Input: dimensioned drawing with shaded views. Units: mm. Origin: part minimum x, y, z. A direction names the side the tool comes from. Give positions to 0.01 mm unless a question says otherwise; leave off trailing zeros. Write each loop counter-clockwise with the first axis right and the second up, starting at its lowest first coordinate (ties: lowest second). Pieces come first, ordered by that corner, then holes.
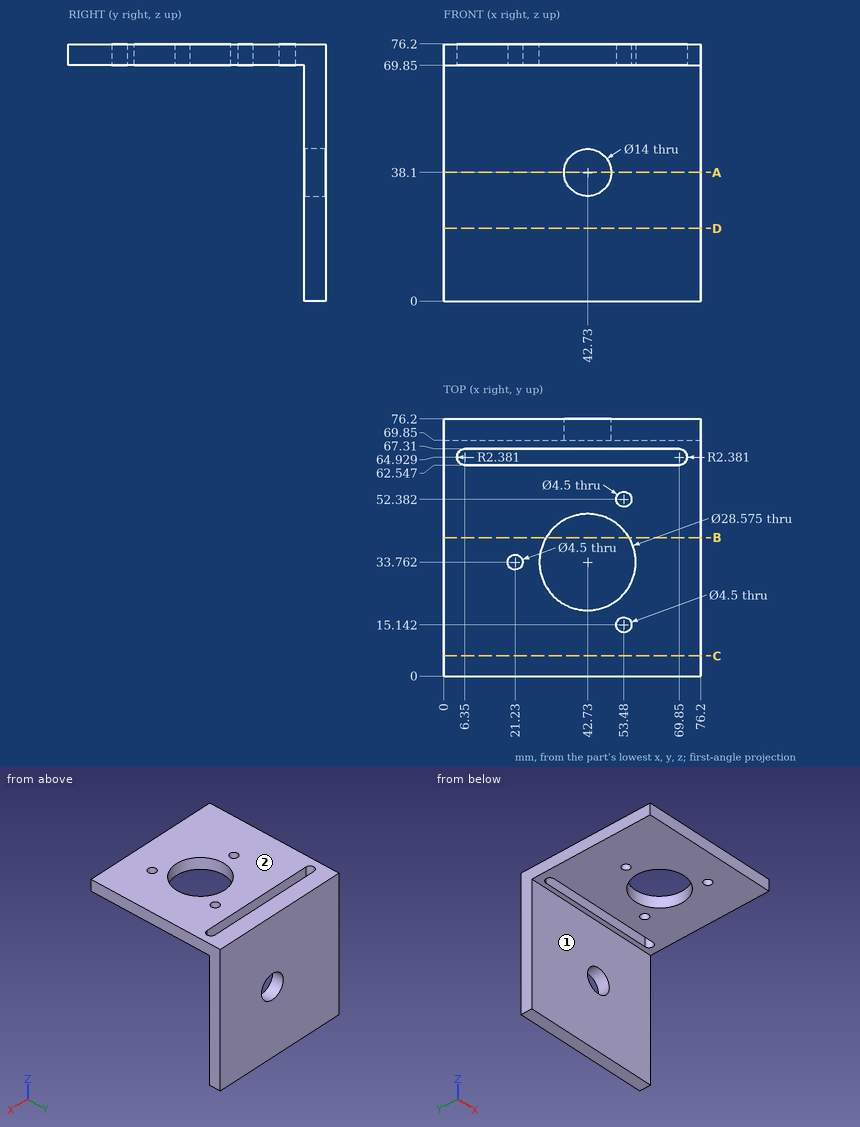
Item 1: Section A-A, the plane z = 38.1. Return the cut outline in (x, y), plus the area to 3 significant figures.
Found:
outline: (0, 69.85) - (35.73, 69.85) - (35.73, 76.2) - (0, 76.2) - close; (49.73, 69.85) - (76.2, 69.85) - (76.2, 76.2) - (49.73, 76.2) - close
area: 395 mm2
Item 2: Section B-B, the plane y = 41. Return the cut outline in (x, z).
Found:
outline: (0, 69.85) - (30.41, 69.85) - (30.41, 76.2) - (0, 76.2) - close; (55.05, 69.85) - (76.2, 69.85) - (76.2, 76.2) - (55.05, 76.2) - close
Item 3: Section C-C, the plane y = 6. Return the cut outline in (x, z).
Found:
outline: (0, 69.85) - (76.2, 69.85) - (76.2, 76.2) - (0, 76.2) - close
Item 4: Reachability of the marked faces 1 and 2 from +Z, -Z, +X, -X, +Y, -Y: full face, straight path, thin tool, end or side. Return the list, or none.
Found:
face 1: -Z, +X, -X, -Y
face 2: +Z, +X, -X, +Y, -Y
Item 5: Line query: L1, parallel to X at y = 71, z = 38; L2, parallel to Y at x = 73, z = 47. Output: solid intervals per line, ascending.
Found:
L1: x = 0 to 35.73, 49.73 to 76.2
L2: y = 69.85 to 76.2
Item 6: Pin query (flat end, axial travel): pin 1 Ø4 at (x, y) = (34, 20.5) entering from -Z; pin 2 Ø2 at (x, y) = (9.5, 65.5) entering from -Z; pin 3 Ø1 at (x, z) = (12, 67.5) entering from -Y; pin 4 Ø5 at (x, y) = (21.23, 33.76) entering from +Z. Return the tip coordinate at first contact, or that it passes through.
Found:
pin 1: stops at z = 69.85
pin 2: passes through
pin 3: stops at y = 69.85
pin 4: stops at z = 76.2
